from build123d import *

# Parameters (mm, degrees)
SKETCH1_W                        = 254
SKETCH1_H                        = 254
BOSS_EXTRUDE1_DEPTH              = 9.525
SKETCH7_W                        = 9.525
SKETCH7_H                        = 38.1
CUT_EXTRUDE4_DEPTH               = 180.857514786
F_10_0_1935_DIAMETER_HOLE1_D     = 4.9149
F_10_0_1935_DIAMETER_HOLE1_DEPTH = 12.7
F_10_0_1935_DIAMETER_HOLE1_TIP   = 1.476584928
F_10_0_1935_DIAMETER_HOLE3_D     = 4.9149
F_10_0_1935_DIAMETER_HOLE3_DEPTH = 12.7
F_10_0_1935_DIAMETER_HOLE3_TIP   = 1.476584928
SKETCH16_W                       = 254
SKETCH16_H                       = 101.6
CUT_EXTRUDE5_DEPTH               = 180.857514786


with BuildPart() as part:
    # Sketch1 → Boss-Extrude1 (new body)
    with BuildSketch(Plane(origin=(0, 0, 0), x_dir=(1, 0, 0), z_dir=(0, 1, 0))):
        Rectangle(SKETCH1_W, SKETCH1_H)
    extrude(amount=BOSS_EXTRUDE1_DEPTH)

    # Sketch7 → Cut-Extrude4 (cut, through all)
    with BuildSketch(Plane(origin=(0, 9.525, 0), x_dir=(1, 0, 0), z_dir=(0, 1, 0))):
        with Locations((-122.2375, 25.4)):
            Rectangle(SKETCH7_W, SKETCH7_H)
        with Locations((122.2375, 25.4)):
            Rectangle(SKETCH7_W, SKETCH7_H)
    extrude(amount=-CUT_EXTRUDE4_DEPTH, mode=Mode.SUBTRACT)

    # #10 (0.1935) Diameter Hole1
    with Locations(Plane(origin=(117.475, 0, 0), x_dir=(0, 0, -1), z_dir=(1, 0, 0))):
        with Locations((11.1125, 4.7625), (39.6875, 4.7625)):
            Hole(F_10_0_1935_DIAMETER_HOLE1_D / 2, depth=F_10_0_1935_DIAMETER_HOLE1_DEPTH)
            with Locations((0, 0, -(F_10_0_1935_DIAMETER_HOLE1_DEPTH + F_10_0_1935_DIAMETER_HOLE1_TIP / 2))):  # 118° drill point
                Cone(0, F_10_0_1935_DIAMETER_HOLE1_D / 2, F_10_0_1935_DIAMETER_HOLE1_TIP, mode=Mode.SUBTRACT)

    # #10 (0.1935) Diameter Hole3
    with Locations(Plane.ZY.offset(117.475)):
        with Locations((-39.6875, 4.7625), (-11.1125, 4.7625)):
            Hole(F_10_0_1935_DIAMETER_HOLE3_D / 2, depth=F_10_0_1935_DIAMETER_HOLE3_DEPTH)
            with Locations((0, 0, -(F_10_0_1935_DIAMETER_HOLE3_DEPTH + F_10_0_1935_DIAMETER_HOLE3_TIP / 2))):  # 118° drill point
                Cone(0, F_10_0_1935_DIAMETER_HOLE3_D / 2, F_10_0_1935_DIAMETER_HOLE3_TIP, mode=Mode.SUBTRACT)

    # Sketch16 → Cut-Extrude5 (cut, through all)
    with BuildSketch(Plane(origin=(0, 9.525, 0), x_dir=(1, 0, 0), z_dir=(0, 1, 0))):
        with Locations((0, -76.2)):
            Rectangle(SKETCH16_W, SKETCH16_H)
    extrude(amount=-CUT_EXTRUDE5_DEPTH, mode=Mode.SUBTRACT)


solid = part.part
Part model, mm, in its own coordinate system. A direction names the side the tool comes from. Coordinates: 2 decimals unless noted, no trailing zeros. Write each loop counter-clockwise with the first axis right and the second up, starting at its lowest first coordinate (ties: lowest second). Pieces come first, ordered by that corner, then holes. Notation, with made-up numbers: M 70.25,-39 L 114.25,-39 A24 ccw 114.25,-19 Z; hole C 33,1.5 d6. An arc over 180 degrees is marked long. Return JSON: item names as keys, results as strings.
1. Saw through at B-B, the plane z = -23.5. Write the cut outline in (x, y) (3 decimals).
Determined:
{"outline": "M -117.475,0 L 117.475,0 L 117.475,9.525 L -117.475,9.525 Z"}
2. Probe L1, parallel to X at y = 0.5, z = -40 (3 decimals). List the from-to ranges inside material, lowest first.
Determined:
{"L1": "-117.475 to 117.475"}
3. Pull direction Y, two halves, no side cores. Call faces 4 (the face through (-2, 9.525, -52)), 5 (the face through (-127, 5, -85)), 6 (the face through (-2, 0, -52)), 7 (the face through (-103.555, 4.781, -40.114)): pulls with the +Y half, pulls with the -Y half, needs draft (parallel to the pull), parting line crosses it, or undercut.
Determined:
{"face 4": "pulls with the +Y half", "face 5": "needs draft", "face 6": "pulls with the -Y half", "face 7": "undercut"}
4. Flat gauge pins, fed straight in: pin 1 Ø4.5 at (y, z) = (4.76, -11.11) entering from -X; pin 2 Ø3 at (y, z) = (4.76, -11.11) entering from -X; pin 3 Ø5 at (y, z) = (4.5, -32.5) entering from +X (3 decimals). Where does each tip first touch, or does it go through?
Determined:
{"pin 1": "x = -104.65", "pin 2": "x = -104.2", "pin 3": "x = 117.475"}
5. 3-axis set-ups, long thin cutter, end or side, ignore diameter. For faces 1 (the face through (111.04, 3.27, -41.64)), 2 (the face through (117.475, 5, -25)), 3 (the face through (-111.04, 3.27, -9.16)): which of +Z, -Z, +X, -X, +Y, -Y reach the whole face in a straight line?
Determined:
{"face 1": "+X", "face 2": "+X, +Y, -Y", "face 3": "-X"}
6. Saw through at A-A, the plane x = 108.5. Write the cut outline in (y, z) (1 decimal).
Determined:
{"outline": "M 0,-127 L 9.5,-127 L 9.5,25.4 L 0,25.4 Z; hole C 4.8,-39.7 d4.9; hole C 4.8,-11.1 d4.9"}
